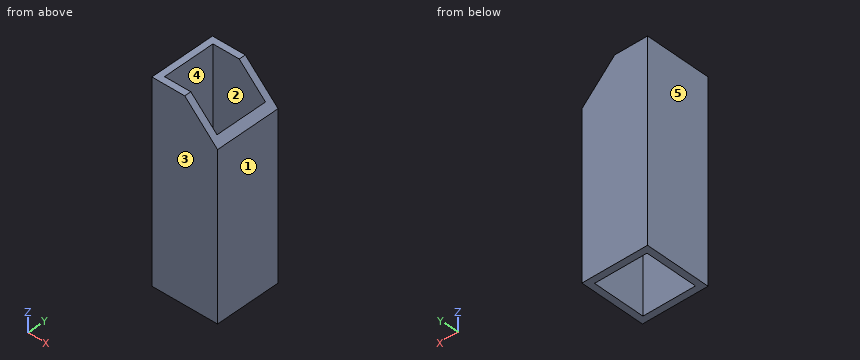
from build123d import *

# Parameters (mm, degrees)
SKETCH2_W           = 50
SKETCH2_H           = 50
SKETCH2_W_2         = 40
SKETCH2_H_2         = 40
BOSS_EXTRUDE1_DEPTH = 150
CUT_EXTRUDE1_DEPTH  = 161.078105936


with BuildPart() as part:
    # Sketch2 → Boss-Extrude1 (new body)
    with BuildSketch(Plane(origin=(0, 0, 0), x_dir=(1, 0, 0), z_dir=(0, 0, -1))):
        Rectangle(SKETCH2_W, SKETCH2_H)
        Rectangle(SKETCH2_W_2, SKETCH2_H_2, mode=Mode.SUBTRACT)
    extrude(amount=-BOSS_EXTRUDE1_DEPTH)

    # Sketch3 → Cut-Extrude1 (cut, through all)
    with BuildSketch(Plane.XZ.offset(25)):
        Polygon((0, 150), (25, 125), (25, 150), align=None)
    extrude(amount=-CUT_EXTRUDE1_DEPTH, mode=Mode.SUBTRACT)


solid = part.part
Geometry: final body of the model. Coordinates: model frame, mm. Face numbers are marked on the shaded views. A direction names the side the tool comes from. Round coordinates to 2 decimals unless told otherwise and drop trailing zeros. Order: outer loops, then holes, each group sorted by start corner. A loop starts at its lowest first (then second) coordinate and runs counter-clockwise, first axis right, second up. Notation, with made-up numbers: (-3.75, 36.25) - (7.25, 36.25) arc R26 ccw to (7.25, 50.25) - close; hole circle Ø10 at (51.5, -8). An arc over 180 degrees is marked (long way). Write each question's results on one line, items separated by ' | '.
Item 1: Section C-C, the plane z = 36. Return the cut outline in (x, y), and give its area (3 significant figures).
Completed:
outline: (-25, -25) - (25, -25) - (25, 25) - (-25, 25) - close; hole (-20, -20) - (20, -20) - (20, 20) - (-20, 20) - close | area: 900 mm^2
Item 2: Mould query, pull axis X, two halves, no side actions, for the marked faces 1, 2 and 3. Classes: pulls with the +X half, pulls with the -X half, needs draft (parallel to the pull), parting line crosses it, or undercut.
Completed:
face 1: pulls with the +X half | face 2: undercut | face 3: needs draft
Item 3: Reachability of the marked faces 4 and 5 from +Z, -Z, +X, -X, +Y, -Y: full face, straight path, thin tool, end or side. Return the list, or none.
Completed:
face 4: +Z, -Z | face 5: +Z, -Z, -X, +Y, -Y
Item 4: Material intervals for line 1 along X through (y, z) = (4.5, 72); line 2 along X through (y, z) = (-3.5, 131), sorted ascending. Write a range as [from, to].
Completed:
line 1: [-25, -20], [20, 25] | line 2: [-25, -20]
Item 5: Section A-A, the plane y = -3. Return the cut outline in (x, z).
Completed:
outline: (-25, 0) - (-20, 0) - (-20, 150) - (-25, 150) - close; (20, 0) - (25, 0) - (25, 125) - (20, 130) - close
Item 6: Section B-B, the plane x = 1.5. Return the cut outline in (y, z).
Completed:
outline: (-25, 0) - (-20, 0) - (-20, 148.5) - (-25, 148.5) - close; (20, 0) - (25, 0) - (25, 148.5) - (20, 148.5) - close
